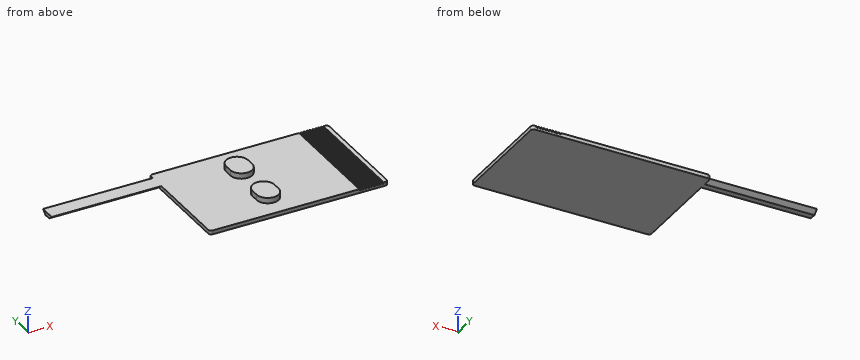
from build123d import *

# Parameters (mm, degrees)
SKETCH_W     = 130
SKETCH_H     = 80
PAD_DEPTH    = 2.85
PAD001_DEPTH = 4
PAD002_DEPTH = 80
FILLET_R     = 2
SKETCH003_W  = 1.05
SKETCH003_H  = 80
POCKET_DEPTH = 1.05


with BuildPart() as part:
    # Sketch → Pad (new body)
    with BuildSketch(Plane.XY):
        Rectangle(SKETCH_W, SKETCH_H)
    extrude(amount=PAD_DEPTH)

    # Sketch001 (on Face6 of Pad) → Pad001 (join)
    with BuildSketch(Plane.XY.offset(2.85)):
        with BuildLine():
            ThreePointArc((-20, 14.75), (-12, 6.75), (-4, 14.75))
            Line((-4, 20.25), (-4, 14.75))
            ThreePointArc((-4, 20.25), (-11.999999, 28.250003), (-20, 20.250002))
            Line((-20, 20.250002), (-20, 14.75))
        make_face()
        with BuildLine():
            ThreePointArc((-20, -20.25), (-12, -28.25), (-4, -20.25))
            Line((-4, -14.75), (-4, -20.25))
            ThreePointArc((-4, -14.75), (-12, -6.75), (-20, -14.75))
            Line((-20, -14.75), (-20, -20.25))
        make_face()
    extrude(amount=PAD001_DEPTH)

    # Sketch002 (on Face2 of Pad001) → Pad002 (join)
    with BuildSketch(Plane(origin=(-65, 0, 0), x_dir=(0, -1, 0), z_dir=(-1, 0, 0))):
        Polygon((-35.765375, 2.85), (-24.265375, 2.85), (-27.715375, 0), (-32.315375, 0), align=None)
    extrude(amount=PAD002_DEPTH)

    # Fillet
    fillet_edges = [part.edges().sort_by_distance(p)[0] for p in [
        (-65, -40, 1.425),
        (65, -40, 1.425),
        (65, 40, 1.425),
        (-65, 40, 1.425),
    ]]
    fillet(fillet_edges, radius=FILLET_R)

    # Sketch003 (on Face5 of Fillet) → Pocket (cut)
    with BuildSketch(Plane.XY.offset(2.85)):
        with Locations((44.525, 0)):
            Rectangle(SKETCH003_W, SKETCH003_H)
        with Locations((46.616892, 0)):
            Rectangle(SKETCH003_W, SKETCH003_H)
        with Locations((48.708784, 0)):
            Rectangle(SKETCH003_W, SKETCH003_H)
        with Locations((50.800676, 0)):
            Rectangle(SKETCH003_W, SKETCH003_H)
        with Locations((52.892568, 0)):
            Rectangle(SKETCH003_W, SKETCH003_H)
        with Locations((54.98446, 0)):
            Rectangle(SKETCH003_W, SKETCH003_H)
        with Locations((57.076352, 0)):
            Rectangle(SKETCH003_W, SKETCH003_H)
        with Locations((59.168244, 0)):
            Rectangle(SKETCH003_W, SKETCH003_H)
        with Locations((61.260136, 0)):
            Rectangle(SKETCH003_W, SKETCH003_H)
    extrude(amount=-POCKET_DEPTH, mode=Mode.SUBTRACT)


solid = part.part
For this review, take the finished solid that the model builds, in its own axes (mm). Give positions to 0.01 mm unless a question says otherwise; leave off trailing zeros. Order: outer loops, then holes, each group sorted by start corner. A loop starts at its lowest first (then second) coordinate and runs counter-clockwise, first axis right, second up. Notation, with made-up numbers: (-7.75, 85) - (20.25, 85) arc R13 ccw to (20.25, 94) - close; hole circle Ø6 at (49.25, -11). An arc over 180 degrees is marked (long way). Answer as a JSON object with one key per item and string values. Group by question number.
Item 1: Clearance check with flat-ended pins moving along their axes: pin 1 Ø3 at (x, z) = (-120, 4.5) entering from +Y; pin 2 Ø1.2 at (y, z) = (18.5, 6) entering from -X; pin 3 Ø4 at (y, z) = (-22, 1.5) entering from -X; pin 4 Ø1.1 at (x, y) = (48, -6) entering from +Z. State where each tip first meets the part, or that it passes through.
Item 2: Take a section at C-C on x = -45. Give the boundary of the cut face in (y, z).
Item 3: Wall thickness on line 1 along Z through (x, y) = (7, 7.5); line 2 along X through (y, z) = (10.5, 1); line 3 along X through (y, z) = (17, 6): over which ranges is each line inside the solid? List them lowest first.
Item 4: Take a section at B-B on x = -12. Give the boundary of the cut face in (y, z), and give its area (3 significant figures).
Item 5: Take a section at A-A on z = 5.75. Give the boundary of the cut face in (x, y).
Item 6: Take a section at D-D on x = -70.5. Give the boundary of the cut face in (y, z).
Reported:
{
 "1": {"pin 1": "through", "pin 2": "x = -20", "pin 3": "x = -65", "pin 4": "z = 2.85"},
 "2": {"outline": "(-40, 0) - (40, 0) - (40, 2.85) - (-40, 2.85) - close"},
 "3": {"line 1": "0 to 2.85", "line 2": "-65 to 65", "line 3": "-20 to -4"},
 "4": {"outline": "(-40, 0) - (40, 0) - (40, 2.85) - (28.25, 2.85) - (28.25, 6.85) - (6.75, 6.85) - (6.75, 2.85) - (-6.75, 2.85) - (-6.75, 6.85) - (-28.25, 6.85) - (-28.25, 2.85) - (-40, 2.85) - close", "area": "400 mm^2"},
 "5": {"outline": "(-20, -20.25) arc R8 ccw to (-4, -20.25) - (-4, -14.75) arc R8 ccw to (-20, -14.75) - close; (-20, 14.75) arc R8 ccw to (-4, 14.75) - (-4, 20.25) arc R8 ccw to (-20, 20.25) - close"},
 "6": {"outline": "(24.27, 2.85) - (27.72, 0) - (32.32, 0) - (35.77, 2.85) - close"}
}
